```python
from build123d import *

# Parameters (mm, degrees)
BOSS_EXTRUDE1_DEPTH     = 40
CUT_EXTRUDE2_DEPTH      = 95.20854526
SKETCH2_4_R             = 12.5
SKETCH2_4_R_2           = 10
BOSS_EXTRUDE2_DEPTH     = 10
CHAMFER1_SIZE           = 10
CUT_EXTRUDE3_DEPTH      = 100.078251902
CUT_EXTRUDE3_DEPTH_BACK = 100.078251902
SKETCH3_R               = 12.5


with BuildPart() as part:
    # Sketch1 → Boss-Extrude1 (new body)
    with BuildSketch(Plane.XY):
        with BuildLine():
            Line((0, 0), (50, 0))
            ThreePointArc((50, 0), (55.303300859, 2.196699141), (57.5, 7.5))
            Line((57.5, 7.5), (57.5, 63))
            Line((57.5, 63), (55, 63))
            Line((55, 63), (55, 7.5))
            ThreePointArc((55, 7.5), (53.535533906, 3.964466094), (50, 2.5))
            Line((50, 2.5), (0, 2.5))
            Line((0, 2.5), (0, 0))
        make_face()
    extrude(amount=-BOSS_EXTRUDE1_DEPTH)

    # Sketch2 → Cut-Extrude2 (cut, through all)
    with BuildSketch(Plane(origin=(57.5, 0, 0), x_dir=(0, 0, -1), z_dir=(1, 0, 0))):
        with BuildLine():
            Line((0, 63), (0, 43.281023868))
            ThreePointArc((0, 43.281023868), (5.956869832, 57.241262542), (20, 63))
            Line((20, 63), (0, 63))
        make_face()
        with BuildLine():
            Line((40, 63), (20, 63))
            ThreePointArc((20, 63), (34.043130168, 57.241262542), (40, 43.281023868))
            Line((40, 43.281023868), (40, 63))
        make_face()
    extrude(amount=-CUT_EXTRUDE2_DEPTH, mode=Mode.SUBTRACT)

    # Sketch2_4 → Boss-Extrude2 (add)
    with BuildSketch(Plane(origin=(57.5, 0, 0), x_dir=(0, 0, -1), z_dir=(1, 0, 0))):
        with Locations((20, 42.997997502)):
            Circle(SKETCH2_4_R)
        with Locations((20, 42.997997502)):
            Circle(SKETCH2_4_R_2, mode=Mode.SUBTRACT)
    extrude(amount=BOSS_EXTRUDE2_DEPTH)

    # Chamfer1
    chamfer1_edges = [part.edges().sort_by_distance(p)[0] for p in [
        (0, 1.25, 0),
        (0, 1.25, -40),
    ]]
    chamfer(chamfer1_edges, length=CHAMFER1_SIZE)

    # Sketch3 → Cut-Extrude3 (cut, two sides: drawn at the far end of the back side and taken through both)
    with BuildSketch(Plane(origin=(0, 2.5, 0), x_dir=(1, 0, 0), z_dir=(0, 1, 0)).offset(-CUT_EXTRUDE3_DEPTH_BACK)):
        with Locations(Location((20, 20, 0), (0, 0, 270))):
            Circle(SKETCH3_R)
    extrude(amount=CUT_EXTRUDE3_DEPTH + CUT_EXTRUDE3_DEPTH_BACK, mode=Mode.SUBTRACT)


solid = part.part
```
Geometry check sheet. Reference: the model listing, model coordinates, mm. A direction names the side the tool comes from. Coordinates: 2 decimals unless noted, no trailing zeros. Order: outer loops, then holes, each group sorted by start corner. A loop starts at its lowest first (then second) coordinate and runs counter-clockwise, first axis right, second up.
Q1. Tool access check on faces 1 (the face through (5, 1, -35)), 2 (the face through (62.43, 46.753, -31.923)), 3 (the face through (36, 2.5, -20)). Record the directions out of +Z, -Z, +X, -X, +Y, -Y that give a thin tool (end or side, any length) a straight path to the whole face; none if there is none.
Reply:
face 1: -Z, -X, +Y, -Y
face 2: +X
face 3: +Z, -Z, -X, +Y
Q2. Sectioned sample at D-D on z = -3.5. Record the cut outline in (x, y).
Reply:
outline: (6.5, 0) - (50, 0) arc R7.5 ccw to (57.5, 7.5) - (57.5, 54.3) - (55, 54.3) - (55, 7.5) arc R5 cw to (50, 2.5) - (6.5, 2.5) - close
Q3. Thickness scan on probe 1 along Y at (x, z) = (62.5, -20); probe 2 along Z at (x, y) = (20, 1); probe 3 along X at (y, z) = (31, -6.5). Record the ranges inside material, lowest first.
Reply:
probe 1: y = 30.5 to 33, 53 to 55.5
probe 2: z = -40 to -32.5, -7.5 to 0
probe 3: x = 55 to 57.5
Q4. Sectioned sample at A-A on x = 20. Record the cut outline in (y, z), and give its area (3 significant figures).
Reply:
outline: (0, -40) - (2.5, -40) - (2.5, -32.5) - (0, -32.5) - close; (0, -7.5) - (2.5, -7.5) - (2.5, 0) - (0, 0) - close
area: 37.5 mm2
Q5. Sectioned sample at C-C on y = 36.5. Record the cut outline in (x, z), and give its area (3 significant figures).
Reply:
outline: (55, -40) - (57.5, -40) - (57.5, -30.68) - (67.5, -30.68) - (67.5, -27.6) - (57.5, -27.6) - (57.5, -12.4) - (67.5, -12.4) - (67.5, -9.32) - (57.5, -9.32) - (57.5, 0) - (55, 0) - close
area: 162 mm2
Q6. Sectioned sample at B-B on z = -15.5. Record the cut outline in (x, y).
Reply:
outline: (0, 0) - (8.34, 0) - (8.34, 2.5) - (0, 2.5) - close; (31.66, 0) - (50, 0) arc R7.5 ccw to (57.5, 7.5) - (57.5, 31.34) - (67.5, 31.34) - (67.5, 34.07) - (57.5, 34.07) - (57.5, 51.93) - (67.5, 51.93) - (67.5, 54.66) - (57.5, 54.66) - (57.5, 62.49) - (55, 62.49) - (55, 7.5) arc R5 cw to (50, 2.5) - (31.66, 2.5) - close
Q7. Depth check by flat-ended pin: pin 1 Ø5 at (x, z) = (58.5, -12.5) entering from -Y; pin 2 Ø12 at (y, z) = (22, -24) entering from -X; pin 3 Ø10 at (x, z) = (58.5, -11.5) entering from -Y. Enter the tip coordinate at first touch or a pass-through.
Reply:
pin 1: stops at y = 3
pin 2: stops at x = 55
pin 3: stops at y = 0.87
Q8. Draft check along Z on faces 4 (the face through (36, 0, -20)), 5 (the face through (44, 1, 0)), 6 (the face through (12.394, 1.233, -29.92)). Enter one of: released by +Z, released by -Z, zero draft, split by the parting line, or undercut.
Reply:
face 4: zero draft
face 5: released by +Z
face 6: undercut
